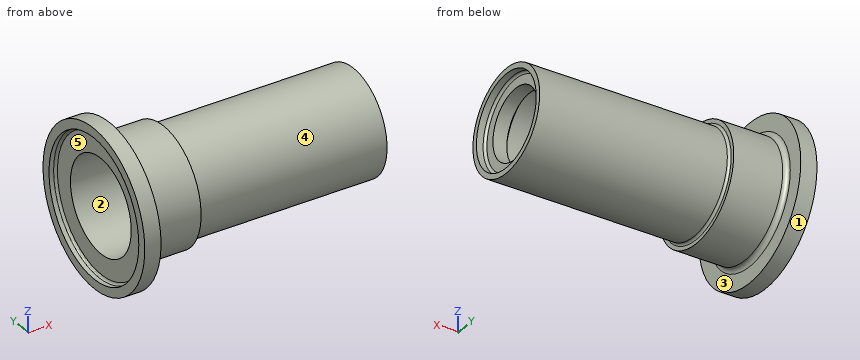
```python
from build123d import *


with BuildPart() as part:
    # Sketch1 → Revolve1 (revolve)
    with BuildSketch(Plane.XY):
        with BuildLine():
            Line((0, 12.5), (0, 11.65))
            ThreePointArc((0, 11.65), (0.146446609, 11.296446609), (0.5, 11.15))
            Line((0.5, 11.15), (40.95, 11.15))
            Line((40.95, 11.15), (40.95, 10))
            Line((40.95, 10), (39.5, 10))
            ThreePointArc((39.5, 10), (39.146446609, 9.853553391), (39, 9.5))
            Line((39, 9.5), (39, 7.5))
            Line((39, 7.5), (36, 7.5))
            Line((36, 7.5), (36, 8.65))
            ThreePointArc((36, 8.65), (35.560660172, 9.710660172), (34.5, 10.15))
            Line((34.5, 10.15), (-13.55, 10.15))
            Line((-13.55, 10.15), (-13.55, 14.5))
            ThreePointArc((-13.55, 14.5), (-13.696446609, 14.853553391), (-14.05, 15))
            Line((-14.05, 15), (-15.05, 15))
            Line((-15.05, 15), (-15.05, 17))
            Line((-15.05, 17), (-11.55, 17))
            Line((-11.55, 17), (-11.55, 13.5))
            ThreePointArc((-11.55, 13.5), (-11.257106781, 12.792893219), (-10.55, 12.5))
            Line((-10.55, 12.5), (0, 12.5))
        make_face()
    revolve(axis=Axis((-88.99, 0, 0), (1, 0, 0)))


solid = part.part
```
Source: CAD feature listing. Evaluate the final solid. Frame: model axes, mm. Face numbers are marked on the shaded views. A direction names the side the tool comes from. Give positions to 0.01 mm unless a question says otherwise; leave off trailing zeros. Write each loop counter-clockwise with the first axis right and the second up, starting at its lowest first coordinate (ties: lowest second). Pieces come first, ordered by that corner, then holes. Notation, with made-up numbers: (-9, 37.25) - (14, 37.25) arc R16 ccw to (14, 41.25) - close; hole circle Ø8 at (23, 39). An arc over 180 degrees is marked (long way). One line per item, written item: value. Start each with the question number.
Q1. Material intervals for probe 1 along Z at (x, y) = (39.9, 0); probe 2 along Z at (x, y) = (38, 0); probe 3 along X at (y, z) = (10.5, 12), sorted ascending. Write a range as from..to.
Q2. Section query B-B, the plane x = 37. Return the cut outline in (y, z).
Q3. Section query A-A, the plane x = 27.5. Return the cut outline in (y, z), then the cut area to 3 significant figures.
Q4. Set-up query: the marked faces 4 and 5. Return all of +Z, -Z, +X, -X, +Y, -Y with unobstructed straight access to the full face (end or side cutting, diameter ignored); none if empty.
Q5. First-contact query: pin 1 Ø12 at (y, z) = (-6.5, -6.5) entering from +X; pin 2 Ø10 at (x, y) = (20, 1.5) entering from +Z; pin 3 Ø1 at (y, z) = (-9, -9.5) entering from -X; pin 4 Ø3 at (x, z) = (6, -3) entering from -Y. Flat tips, straight axial feed; report the tip coordinate or a pass-through.
Q6. Draft query along Z for the marked faces 1, 2 and 3. Return one class per face: +Z half, -Z half, draft (parallel to the pull), parting line (faces both ways), or undercut.
Answer:
1. probe 1: z = -11.15..-10, 10..11.15
1. probe 2: z = -11.15..-7.5, 7.5..11.15
1. probe 3: x = -15.05..-11.55
2. outline: circle Ø22.3 at (0, 0); hole circle Ø15 at (0, 0)
3. outline: circle Ø22.3 at (0, 0); hole circle Ø20.3 at (0, 0)
3. area: 66.9 mm2
4. face 4: +X
4. face 5: -X
5. pin 1: stops at x = 40.95
5. pin 2: stops at z = 11.15
5. pin 3: stops at x = -13.55
5. pin 4: stops at y = -11.05
6. face 1: parting line
6. face 2: undercut
6. face 3: draft
